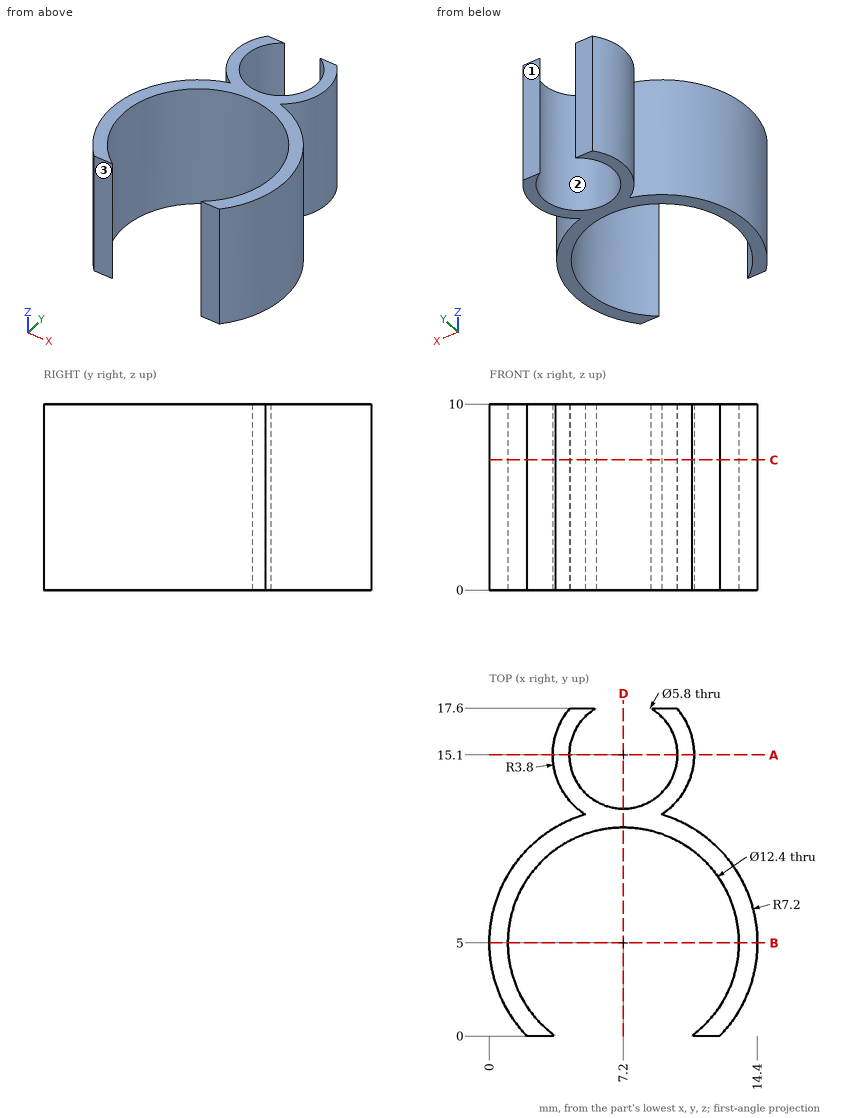
Job drawing, mm, ordinate dimensions from the low corner. One solid piece. Coordinates: 2 decimals unless noted, no trailing zeros. Order: outer loops, then holes, each group sorted by start corner. A loop starts at its lowest first (then second) coordinate and runs counter-clockwise, first axis right, second up. Notation, with made-up numbers: (25, -2) -> (78, -2) arc R21 cw to (78, 8) -> close; hole circle Ø3 at (-17, 73.5). An arc over 180 degrees is marked (long way). Answer in a Markdown table with one row per item. Add a question column.
Q1. Wall check: line 1 along X through (y, z) = (5, 3.75); line 2 along Y through (x, z) = (9.5, 6.75); line 3 along X through (y, z) = (15.1, 8.25). Give the ranges that are in metal, low to high. Write a range as [from, to].
Q2. Drop flat-ended pins along their axis: pin 1 (2 mm diameter, centred on x = 7.5, z = 2, fed in from -Y); pin 2 (3 mm diameter, centred on y = 8.5, z = 7.5, fed in from -X). Give the stop position or say it passes through.
Q3. Band-saw the part on D-D, the plane x = 7.2. List the corners of the cut face in (y, z).
Q4. Mould opens along Y. For the marked faces 1, 2 and 3 say: +Y half, -Y half, draft (parallel to the pull), parting line (faces both ways), or undercut.
Q5. Band-saw the part on A-A, the plane y = 15.1. List the corners of the cut face in (x, z).
Q6. Band-saw the part on B-B, the plane y = 5. List the corners of the cut face in (x, z).
Q7. Band-saw the part on C-C, the plane z = 7. List the corners of the cut face in (x, y).
Answers follow:
| question | item | result |
|---|---|---|
| 1 | line 1 | [0, 1], [13.4, 14.4] |
| 1 | line 2 | [10.76, 11.82], [12.08, 13.33], [16.87, 17.6] |
| 1 | line 3 | [3.4, 4.3], [10.1, 11] |
| 2 | pin 1 | y = 11.06 |
| 2 | pin 2 | x = 0.28 |
| 3 | outline | (11.2, 0) -> (12.2, 0) -> (12.2, 10) -> (11.2, 10) -> close |
| 4 | face 1 | +Y half |
| 4 | face 2 | undercut |
| 4 | face 3 | -Y half |
| 5 | outline | (3.4, 0) -> (4.3, 0) -> (4.3, 10) -> (3.4, 10) -> close; (10.1, 0) -> (11, 0) -> (11, 10) -> (10.1, 10) -> close |
| 6 | outline | (0, 0) -> (1, 0) -> (1, 10) -> (0, 10) -> close; (13.4, 0) -> (14.4, 0) -> (14.4, 10) -> (13.4, 10) -> close |
| 7 | outline | (2.02, 0) -> (3.53, 0) arc R6.2 cw (long way) to (10.87, 0) -> (12.38, 0) arc R7.2 ccw to (9.25, 11.9) arc R3.8 ccw to (10.06, 17.6) -> (8.67, 17.6) arc R2.9 cw (long way) to (5.73, 17.6) -> (4.34, 17.6) arc R3.8 ccw to (5.15, 11.9) arc R7.2 ccw to start |
